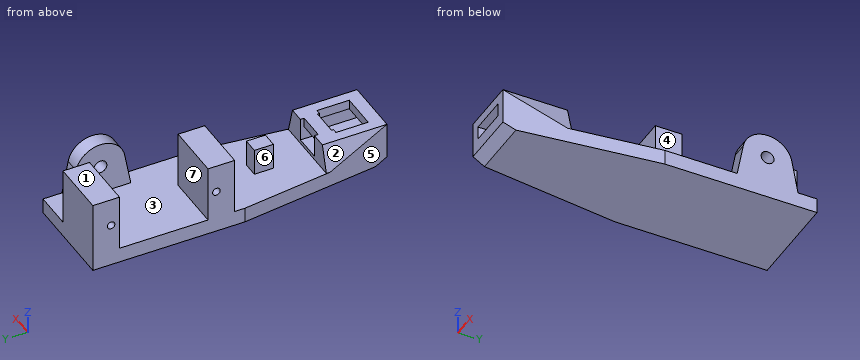
from build123d import *
from OCP.BRepFilletAPI import BRepFilletAPI_MakeChamfer

# Parameters (mm, degrees)
RESSALTO_EXTRUS_O1_DEPTH = 4
ESBO_O2_W                = 15
ESBO_O2_H                = 7
ESBO_O2_W_2              = 4
ESBO_O2_H_2              = 16
RESSALTO_EXTRUS_O2_DEPTH = 15
ESBO_O3_R                = 1
CORTE_EXTRUS_O1_DEPTH    = 84.582294776
ESBO_O10_R               = 1.7
CORTE_EXTRUS_O4_DEPTH    = 10
RESSALTO_EXTRUS_O3_DEPTH = 17
RESSALTO_EXTRUS_O4_REACH = 84.348
ESBO_O7_W                = 4
ESBO_O7_H                = 5
ESBO_O8_W                = 15
ESBO_O8_H                = 3.5
RESSALTO_EXTRUS_O5_DEPTH = 2.5
CHANFRO2_SIZE            = 7
CHANFRO2_SIZE_2          = 2
CHANFRO3_SIZE            = 1.5
CHANFRO3_SIZE2           = 3.216760381


with BuildPart() as part:
    # Esboço1 → Ressalto-extrusão1 (new body)
    with BuildSketch(Plane.XY):
        Polygon((-12.5, 0), (12.5, 0), (12.5, -40), (7.5, -80), (-7.5, -80), (-12.5, -40), align=None)
    extrude(amount=RESSALTO_EXTRUS_O1_DEPTH)

    # Esboço2 → Ressalto-extrusão2 (add)
    with BuildSketch(Plane.XY.offset(4)):
        with Locations((-5, -33.8)):
            Rectangle(ESBO_O2_W, ESBO_O2_H)
        with Locations((-5, -3.5)):
            Rectangle(ESBO_O2_W, ESBO_O2_H)
        with Locations((10.5, -13)):
            Rectangle(ESBO_O2_W_2, ESBO_O2_H_2)
    extrude(amount=RESSALTO_EXTRUS_O2_DEPTH)

    # Esboço3 → Corte-extrusão1 (cut, through all)
    with BuildSketch(Plane(origin=(2.5, 0, 0), x_dir=(0, 0, -1), z_dir=(1, 0, 0))):
        with Locations(Location((-11.5, -4.8, 0), (0, 0, 90))):
            Circle(ESBO_O3_R)
        with Locations(Location((-11.5, -32.5, 0), (0, 0, 90))):
            Circle(ESBO_O3_R)
    extrude(amount=-CORTE_EXTRUS_O1_DEPTH, mode=Mode.SUBTRACT)

    # Esboço10 → Corte-extrusão4 (cut)
    with BuildSketch(Plane(origin=(12.5, 0, 0), x_dir=(0, 0, -1), z_dir=(1, 0, 0))):
        with Locations((-11.5, -13)):
            Circle(ESBO_O10_R)
        with BuildLine():
            Line((-4, -5), (-19, -5))
            Line((-19, -5), (-19, -21))
            Line((-19, -21), (-4, -21))
            Line((-4, -21), (-12.684004699, -19.391254405))
            ThreePointArc((-12.684004699, -19.391254405), (-18, -13), (-12.684004699, -6.608745595))
            Line((-12.684004699, -6.608745595), (-4, -5))
        make_face()
    extrude(amount=-CORTE_EXTRUS_O4_DEPTH, mode=Mode.SUBTRACT)

    # Esboço6 → Ressalto-extrusão3 (add)
    with BuildSketch(Plane.XZ.offset(80)):
        Polygon((-5, 5), (-5, 8.5), (-4.75, 8.5), (-4.75, 11), (-7.5, 11), (-7.5, 4), (7.5, 4), (7.5, 11), (4.75, 11), (4.75, 8.5), (5, 8.5), (5, 5), align=None)
    extrude(amount=-RESSALTO_EXTRUS_O3_DEPTH)

    # Ressalto-extrusão4: up to this face of the body (flat: up to its plane)
    ressalto_extrus_o4_end = Plane(part.part.faces().sort_by_distance((-6.125, -71.5, 11))[0])
    # Esboço7 → Ressalto-extrusão4 (add, up to the picked face)
    with BuildSketch(Plane.XY.offset(4), mode=Mode.PRIVATE) as ressalto_extrus_o4_sk1:
        with Locations((0, -50.5)):
            Rectangle(ESBO_O7_W, ESBO_O7_H)
    ressalto_extrus_o4_tool1 = split(extrude(ressalto_extrus_o4_sk1.sketch, amount=RESSALTO_EXTRUS_O4_REACH, mode=Mode.PRIVATE), bisect_by=ressalto_extrus_o4_end, keep=Keep.BOTH, mode=Mode.PRIVATE)
    # Esboço7 → Ressalto-extrusão4 (add, up to the picked face)
    with BuildSketch(Plane.XY.offset(4), mode=Mode.PRIVATE) as ressalto_extrus_o4_sk2:
        with Locations((5.5, -65.5)):
            Rectangle(ESBO_O7_W, ESBO_O7_H)
    ressalto_extrus_o4_tool2 = split(extrude(ressalto_extrus_o4_sk2.sketch, amount=RESSALTO_EXTRUS_O4_REACH, mode=Mode.PRIVATE), bisect_by=ressalto_extrus_o4_end, keep=Keep.BOTH, mode=Mode.PRIVATE)
    # Esboço7 → Ressalto-extrusão4 (add, up to the picked face)
    with BuildSketch(Plane.XY.offset(4), mode=Mode.PRIVATE) as ressalto_extrus_o4_sk3:
        with Locations((-5.5, -65.5)):
            Rectangle(ESBO_O7_W, ESBO_O7_H)
    ressalto_extrus_o4_tool3 = split(extrude(ressalto_extrus_o4_sk3.sketch, amount=RESSALTO_EXTRUS_O4_REACH, mode=Mode.PRIVATE), bisect_by=ressalto_extrus_o4_end, keep=Keep.BOTH, mode=Mode.PRIVATE)
    add(ressalto_extrus_o4_tool1.solids().sort_by(Axis((0, -50.5, 4), (0, 0, 1)))[0])
    add(ressalto_extrus_o4_tool2.solids().sort_by(Axis((5.5, -65.5, 4), (0, 0, 1)))[0])
    add(ressalto_extrus_o4_tool3.solids().sort_by(Axis((-5.5, -65.5, 4), (0, 0, 1)))[0])

    # Esboço8 → Ressalto-extrusão5 (add)
    with BuildSketch(Plane.XY.offset(11)):
        with Locations((0, -78.25)):
            Rectangle(ESBO_O8_W, ESBO_O8_H)
        with Locations((0, -65.75)):
            Rectangle(ESBO_O8_W, ESBO_O8_H)
    extrude(amount=-RESSALTO_EXTRUS_O5_DEPTH)

    # Chanfro2
    chanfro2_edges_1 = [part.edges().sort_by_distance(p)[0] for p in [
        (7.5, -71.5, 4),
    ]]
    chanfro2_side_1 = [part.faces().sort_by_distance(p)[0] for p in [
        (7.5, -71.5, 4.04),
    ]]
    chanfro2_edges_2 = [part.edges().sort_by_distance(p)[0] for p in [
        (-7.5, -71.5, 4),
    ]]
    chanfro2_side_2 = [part.faces().sort_by_distance(p)[0] for p in [
        (-7.5, -71.5, 4.04),
    ]]
    chanfro2 = BRepFilletAPI_MakeChamfer(part.part.solid().wrapped)
    for e in chanfro2_edges_1:
        chanfro2.Add(CHANFRO2_SIZE - 0.0001, CHANFRO2_SIZE_2 - 0.0001, e.wrapped, chanfro2_side_1[0].wrapped)
    for e in chanfro2_edges_2:
        chanfro2.Add(CHANFRO2_SIZE - 0.0001, CHANFRO2_SIZE_2 - 0.0001, e.wrapped, chanfro2_side_2[0].wrapped)
    add(Compound.cast(chanfro2.Shape()), mode=Mode.REPLACE)  # a hair under: the kernel refuses the full size

    # Chanfro3
    chanfro3_edges = [part.edges().sort_by_distance(p)[0] for p in [
        (0, -80, 0),
    ]]
    chanfro3_side = [part.faces().sort_by_distance(p)[0] for p in [
        (7.313989248, -80, 10.99995),
    ]]
    chamfer(chanfro3_edges, length=CHANFRO3_SIZE, length2=CHANFRO3_SIZE2, reference=chanfro3_side[0])


solid = part.part
Work out the finished part from the listing and answer in its coordinate system (mm). Face numbers are marked on the shaded views. A direction names the side the tool comes from. Round coordinates to 2 decimals unless told otherwise and drop trailing zeros. Loops run counter-clockwise (first coordinate to the right, second up) from the corner with the lowest first, then second, coordinate; pieces in that order, holes last. Notation, with made-up numbers: (-37, 28.25) - (-25, 28.25) arc R18 ccw to (-25, 33.25) - close; hole circle Ø5 at (-14.75, -24.5). An arc over 180 degrees is marked (long way). One line per item, written item: value.
Q1. For the marked faces 1, 2 and 3, determine the directions among +Z, -Z, +X, -X, +Y, -Y from which every point of the face is accessible in a straight line to the end or side of a thin tool.
Check values:
face 1: +Z, +X, -X, +Y, -Y
face 2: +Z, -X, -Y
face 3: +Z
Q2. Find section C-C on z = 14.5. Give the vertices of the cut face in (x, y), and give its area (3 significant figures).
Check values:
outline: (-12.5, -37.3) - (2.5, -37.3) - (2.5, -30.3) - (-12.5, -30.3) - close; (-12.5, -7) - (2.5, -7) - (2.5, 0) - (-12.5, 0) - close; (8.5, -18.77) - (12.5, -18.77) - (12.5, -7.23) - (8.5, -7.23) - close
area: 256 mm2
Q3. Find section D-D on x = 11.25. Give the vertices of the cut face in (y, z).
Check values:
outline: (-50, 0) - (0, 0) - (0, 4) - (-5, 4) - (-6.61, 12.68) arc R6.5 ccw to (-19.39, 12.68) - (-21, 4) - (-50, 4) - close; hole circle Ø3.4 at (-13, 11.5)
Q4. The mould has two halves that part along Y. Classify the marked faces 4, 5, 6 and 7: +Y half, -Y half, draft (parallel to the pull), parting line (faces both ways), or undercut.
Check values:
face 4: draft
face 5: -Y half
face 6: undercut
face 7: undercut
Q5. Straight lines are drawn through the part: probe 1 along Y at (x, z) = (-6, 5); probe 2 along Y at (x, z) = (-2.25, 16.5); probe 3 along Y at (x, z) = (-10.5, 12.25). For each, find the intervals that lie inside material, in ascending order.
Check values:
probe 1: -80 to -63, -37.3 to -30.3, -7 to 0
probe 2: -37.3 to -30.3, -7 to 0
probe 3: -37.3 to -33.16, -31.84 to -30.3, -7 to -5.46, -4.14 to 0
Q6. Find section B-B on x = -6. Give the vertices of the cut face in (y, z).
Check values:
outline: (-80, 1.5) - (-76.78, 0) - (0, 0) - (0, 19) - (-7, 19) - (-7, 4) - (-30.3, 4) - (-30.3, 19) - (-37.3, 19) - (-37.3, 4) - (-63, 4) - (-63, 11) - (-80, 11) - close; hole circle Ø2 at (-32.5, 11.5); hole circle Ø2 at (-4.8, 11.5)
Q7. Find section A-A on y = -13. Give the vertices of the cut face in (x, z).
Check values:
outline: (-12.5, 0) - (12.5, 0) - (12.5, 9.8) - (8.5, 9.8) - (8.5, 4) - (-12.5, 4) - close; (8.5, 13.2) - (12.5, 13.2) - (12.5, 18) - (8.5, 18) - close
Q8. Each of these flat-tipped pins is pushed along its axis until it touches: pin 1 Ø8 at (x, y) = (-2, -68.5) entering from +Z; pin 2 Ø2.5 at (y, z) = (-49.5, 9) entering from +X; pin 3 Ø4 at (y, z) = (-14, 8) entering from -X. Where does it stop, or does it pass through?
Check values:
pin 1: z = 11
pin 2: x = 2
pin 3: x = 8.5
